Part model, mm, in its own coordinate system. A direction names the side the tool comes from. Give positions to 0.01 mm unless a question says otherwise; leave off trailing zeros. Write each loop counter-clockwise with the first axis right and the second up, starting at its lowest first coordinate (ties: lowest second). Pieces come first, ordered by that corner, then holes.
```python
from build123d import *

# Parameters (mm, degrees)
ESQUISSE1_W         = 4
ESQUISSE1_H         = 85
BOSS_EXTRU_1_DEPTH  = 22.93
BOSS_EXTRU_5_DEPTH  = 22.95
CONG_1_R            = 2
ESQUISSE7_W         = 4
ESQUISSE7_H         = 21.820353027
BOSS_EXTRU_10_DEPTH = 25.35
CONG_14_R           = 1
CONG_15_R           = 1
BOSS_EXTRU_11_DEPTH = 1
BOSS_EXTRU_12_DEPTH = 22.95


with BuildPart() as part:
    # Esquisse1 → Boss.-Extru.1 (new body)
    with BuildSketch(Plane.XY):
        with Locations((-2, -15.95097561)):
            Rectangle(ESQUISSE1_W, ESQUISSE1_H)
    extrude(amount=BOSS_EXTRU_1_DEPTH)

    # Esquisse2 → Boss.-Extru.5 (add)
    with BuildSketch(Plane.XY.offset(22.93)):
        Polygon((-32.681935281, 38.444276031), (0, 26.54902439), (0, 22.54902439), (-4, 22.54902439), (-34.435421614, 33.626611925), align=None)
    extrude(amount=-BOSS_EXTRU_5_DEPTH)

    # Congé1
    cong_1_edges = [part.edges().sort_by_distance(p)[0] for p in [
        (-2, -58.45097561, 22.93),
        (-2, -58.45097561, 0),
    ]]
    fillet(cong_1_edges, radius=CONG_1_R)

    # Esquisse7 → Boss.-Extru.10 (add)
    with BuildSketch(Plane(origin=(0, 0, 0), x_dir=(0, 0, -1), z_dir=(1, 0, 0))):
        with Locations((-2, -32.381152124)):
            Rectangle(ESQUISSE7_W, ESQUISSE7_H)
    extrude(amount=-BOSS_EXTRU_10_DEPTH)

    # Congé14
    cong_14_edges = [part.edges().sort_by_distance(p)[0] for p in [
        (-25.35, -43.291328637, 2),
        (-25.35, -21.47097561, 2),
    ]]
    fillet(cong_14_edges, radius=CONG_14_R)

    # Congé15
    cong_15_edges = [part.edges().sort_by_distance(p)[0] for p in [
        (-14.175, -43.291328637, 0),
        (-25.35, -32.381152123, 0),
        (-14.175, -21.47097561, 0),
        (-25.057106781, -21.763868829, 0),
        (-25.057106781, -42.998435418, 0),
    ]]
    fillet(cong_15_edges, radius=CONG_15_R)

    # Esquisse10 → Boss.-Extru.11 (add)
    with BuildSketch(Plane.ZY.offset(4)):
        Polygon((7.751431337, 10.464501792), (12.751431337, 10.464501792), (12.751431337, 15.464501792), (10.751431337, 15.464501792), (10.751431337, 12.464501792), (7.751431337, 12.464501792), align=None)
    extrude(amount=BOSS_EXTRU_11_DEPTH)

    # Esquisse13 → Boss.-Extru.12 (add)
    with BuildSketch(Plane.XY):
        Polygon((-5.151966744, 23.320636857), (-3.656231692, 20.681104413), (-2.075100003, 23.320636857), align=None)
    extrude(amount=BOSS_EXTRU_12_DEPTH)


solid = part.part
```
1) 3-axis set-ups, long thin cutter, end or side, ignore diameter. For faces 1 (the face through (-14, -21.471, 3)), 2 (the face through (-15, -33, 4)), 3 (the face through (-17, 29, -0.02)), 4 (the face through (-4, 22, 22.95)), 5 (the face through (-5, 12, 11)): which of +Z, -Z, +X, -X, +Y, -Y reach the whole face in a straight line?
Answers follow:
face 1: +Z, -Z, -X
face 2: +Z, -X, -Y
face 3: -Z, +X, -X, +Y, -Y
face 4: +Z, +X, -X, +Y, -Y
face 5: +Z, -Z, -X, -Y
2) Saw through at C-C, the plane z = 9. Write the cut outline in (x, y), then the cut area to 3 significant figures.
Answers follow:
outline: (-34.44, 33.63) - (-4.9, 22.88) - (-4, 21.29) - (-4, 12.46) - (-5, 12.46) - (-5, 10.46) - (-4, 10.46) - (-4, -58.45) - (0, -58.45) - (0, 26.55) - (-32.68, 38.44) - close
area: 507 mm2
3) Saw through at B-B, the plane x = -21.5. Write the cut outline in (y, z).
Answers follow:
outline: (-43.29, 1) arc R1 ccw to (-42.29, 0) - (-22.47, 0) arc R1 ccw to (-21.47, 1) - (-21.47, 4) - (-43.29, 4) - close; (28.92, -0.02) - (34.37, -0.02) - (34.37, 22.93) - (28.92, 22.93) - close
4) Saw through at A-A, the plane y = -25.5. Write the cut outline in (x, z), then the cut area to 3 significant figures.
Answers follow:
outline: (-25.35, 1) arc R1 ccw to (-24.35, 0) - (0, 0) - (0, 22.93) - (-4, 22.93) - (-4, 4) - (-25.35, 4) - close
area: 177 mm2
5) Pin check, flat tips, straight feed: pin 1 Ø1.5 at (x, z) = (-15.5, 2) entering from -Y; pin 2 Ø1.1 at (x, z) = (-4.5, 11.5) entering from +Y; pin 3 Ø2.5 at (x, z) = (-16, 3) entering from +Y. Stop position of each tip, or through.
Answers follow:
pin 1: stops at y = -43.29
pin 2: stops at y = 28.39
pin 3: stops at y = 32.83
6) Two-plate mould, pull along Y, no slides. Class faces 6 (the face through (-4, -19, 11)), 7 (the face through (0, -15, 12)), 8 (the face through (-1.97, -57.85, 22.36)): +Y half, -Y half, draft (parallel to the pull), parting line (faces both ways), or undercut.
Answers follow:
face 6: undercut
face 7: draft
face 8: -Y half
7) Wall check: L1, parallel to X at y = -44.5, z = 10; L2, parallel to Z at x = -29, y = 33.5; L3, parallel to Z at x = -19.5, y = -37.5. Give the ranges that are in metal, low to high.
Answers follow:
L1: x = -4 to 0
L2: z = -0.02 to 22.93
L3: z = 0 to 4
8) Saw through at D-D, the plane x = -26.5. Write the cut outline in (y, z).
Answers follow:
outline: (30.74, -0.02) - (36.19, -0.02) - (36.19, 22.93) - (30.74, 22.93) - close
